Check sheet for the modelled part. Datum: model origin and axes. Units: mm. A direction names the side the tool comes from. Round coordinates to 2 decimals unless told otherwise and drop trailing zeros. Write each loop counter-clockwise with the first axis right and the second up, starting at its lowest first coordinate (ties: lowest second). Pieces come first, ordered by that corner, then holes. Notation, with made-up numbers: (4, 20.5) - (49, 20.5) arc R18 ccw to (49, 44.5) - close; hole circle Ø3 at (16.25, 84.25). An arc over 180 degrees is marked (long way). Answer as a JSON object with one key per item and string values. Group by question number.
Item 1: Release check for a two-part mould opening along X. For faces 6 (the flat face through (-25.394, 2.535, -174.72)), 7 (the flat face through (25.575, 2.636, -364.787)), 8 (the flat face through (0, -10, -289)) record: pulls with the +X half, pulls with the -X half, needs draft (parallel to the pull), parting line crosses it, or undercut.
Item 2: Set-up check for faces 1 (the flat face through (25.394, -2.535, -174.72)), 2 (the flat face through (-25.46, -2.47, -174.72)), 3 (the flat face through (25.46, 2.47, -174.72)), 4 (the flat face through (-25.575, -2.636, -364.787)), 5 (the flat face through (0, 5, -175)): record each of +Z, -Z, +X, -X, +Y, -Y from which the full face is reachable in a straight line by a thin tool's end or side.
Item 3: Gauge pin test, flat ends, axial feed: P1, Ø8, axis at y = 6.5, z = -195.5, coming from the +X side; P2, Ø4, axis at y = 0, z = -200, coming from the +X side; P3, Ø3, axis at y = 4, z = -189, coming from the +X side. Record the tip position at first contact, or that the pin passes through.
Item 4: Sectioned sample at B-B on x = -16.5. Record the boundary of the cut face in (y, z).
Item 5: Sectioned sample at D-D on y = 7.25. Record the boundary of the cut face in (x, z), plus the area to 3 significant figures.
Item 6: Sectioned sample at C-C on z = -199.5. Record the boundary of the cut face in (x, y), plus the area to 3 significant figures.
Item 7: Sectioned sample at A-A on z = -171.5. Record the boundary of the cut face in (x, y), plus the area to 3 significant figures.
Item 8: Thickness scan on line 1 (Y direction, x = 0, z = -198); line 2 (Y direction, x = 0, z = -193); line 3 (Z direction, x = 15, y = -1.75). Record the ranges inside material, lowest first.
```python
from build123d import *

# Parameters (mm, degrees)
EXTRUDE_1_DEPTH          = 18
CHAMFER_1_SIZE           = 5
CHAMFER_2_SIZE           = 5
CUT_EXTRUDE_1_DEPTH      = 8
EXTRUDE_2_REACH          = 696.741
EXTRUDE_2_END_RADIUS     = 240
EXTRUDE_3_DEPTH          = 5
EXTRUDE_4_REACH          = 929.644
EXTRUDE_4_END_RADIUS     = 232
SKETCH_10_R              = 12
CUT_EXTRUDE_7_DEPTH      = 695.872110635
CUT_EXTRUDE_7_DEPTH_BACK = 695.872110635
SKETCH_16_OUTSIDE_W      = 362.68
SKETCH_16_OUTSIDE_H      = 1204.68
SKETCH_16_OUTSIDE_W_2    = 100
SKETCH_16_OUTSIDE_H_2    = 230
SKETCH_21_R              = 1.9
CUT_EXTRUDE_17_DEPTH     = 233.862620444
SKETCH_34_OUTSIDE_W      = 120.25
SKETCH_34_OUTSIDE_H      = 70.25
CUT_EXTRUDE_18_DEPTH     = 40
CUT_EXTRUDE_19_DEPTH     = 41


with BuildPart() as part:
    # Sketch 4 → Loft 1 section 0
    with BuildSketch(Plane(origin=(0, 10, 0), x_dir=(1, 0, 0), z_dir=(0, 1, 0))):
        with BuildLine():
            Line((25, 0), (-25, 0))
            Line((-25, 0), (-25, 630))
            Line((-25, 630), (0, 672.857142857))
            Line((0, 672.857142857), (25, 630))
            Line((25, 630), (25, 0))
        make_face()
    # Sketch 1 → Loft 1 section 1
    with BuildSketch(Plane(origin=(0, 0, 0), x_dir=(1, 0, 0), z_dir=(0, 1, 0))):
        with BuildLine():
            Line((-35, 0), (35, 0))
            Line((35, 0), (35, 630))
            Line((35, 630), (0, 690))
            Line((0, 690), (-35, 630))
            Line((-35, 630), (-35, 0))
        make_face()
    loft_1 = loft()

    # Mirror 1: Loft 1 across plane
    add(loft_1.mirror(Plane.ZX))



with BuildPart() as body_2:
    # Sketch 5 → Extrude 1 (new, symmetric)
    with BuildSketch(Plane(origin=(0, 0, 0), x_dir=(1, 0, 0), z_dir=(0, 1, 0))):
        with BuildLine():
            ThreePointArc((-66.346774613, -65.189169183), (0, -55.5), (66.346774613, -65.189169183))
            ThreePointArc((66.346774613, -65.189169183), (73.061224406, -64.270510235), (76.791165228, -58.612302768))
            ThreePointArc((76.791165228, -58.612302768), (79, -30.5), (76.791165228, -2.387697232))
            ThreePointArc((76.791165228, -2.387697232), (0, -15.004503167), (-76.791165228, -2.387697232))
            ThreePointArc((-76.791165228, -2.387697232), (-79, -30.5), (-76.791165228, -58.612302768))
            ThreePointArc((-76.791165228, -58.612302768), (-73.061224406, -64.270510235), (-66.346774613, -65.189169183))
        make_face()
    extrude(amount=EXTRUDE_1_DEPTH, both=True)

    # Chamfer 1
    chamfer_1_edges = [body_2.edges().sort_by_distance(p)[0] for p in [
        (0, 18, 15.004503167),
        (-79, 18, 30.5),
        (-73.061224406, 18, 64.270510235),
        (0, 18, 55.5),
        (73.061224406, 18, 64.270510235),
        (0, -18, 55.5),
        (-73.061224406, -18, 64.270510235),
        (-79, -18, 30.5),
        (79, -18, 30.5),
        (73.061224406, -18, 64.270510235),
        (79, 18, 30.5),
    ]]
    chamfer(chamfer_1_edges, length=CHAMFER_1_SIZE)

    # Chamfer 2
    chamfer_2_edges = [body_2.edges().sort_by_distance(p)[0] for p in [
        (0, -18, 15.004503167),
    ]]
    chamfer(chamfer_2_edges, length=CHAMFER_2_SIZE)

    # Sketch 6 → Cut-Extrude 1 (cut)
    with BuildSketch(Plane(origin=(0, 18, 0), x_dir=(1, 0, 0), z_dir=(0, 1, 0))):
        with BuildLine():
            ThreePointArc((67.221840199, -55.023712607), (68.932610365, -35.286223394), (68.335500378, -15.483731767))
            ThreePointArc((68.335500378, -15.483731767), (0, -25.004503167), (-68.335500378, -15.483731767))
            ThreePointArc((-68.335500378, -15.483731767), (-68.932610365, -35.286223394), (-67.221840199, -55.023712607))
            ThreePointArc((-67.221840199, -55.023712607), (0, -45.5), (67.221840199, -55.023712607))
        make_face()
    cut_extrude_1 = extrude(amount=-CUT_EXTRUDE_1_DEPTH, mode=Mode.SUBTRACT)

    # Mirror 2: Cut-Extrude 1 across plane
    add(cut_extrude_1.mirror(Plane.ZX), mode=Mode.SUBTRACT)


with BuildPart() as part_1:
    add(part.part)

    add(body_2.part)  # Extrude 2 merges body 2
    # Extrude 2: up to this cylinder (the profile starts inside it)
    extrude_2_end = Plane(origin=(0, 0, -224.995496833), z_dir=(0, -1, 0)) * Cylinder(EXTRUDE_2_END_RADIUS, 1874.482, mode=Mode.PRIVATE)
    # Sketch 7 → Extrude 2 (add, up to the surface)
    with BuildSketch(Plane.XY, mode=Mode.PRIVATE) as extrude_2_sk1:
        Polygon((-25.828427125, 12), (-37.828427125, 0), (-25.828427125, -12), (25.828427125, -12), (37.828427125, 0), (25.828427125, 12), align=None)
    extrude_2_tool1 = extrude(extrude_2_sk1.sketch, amount=EXTRUDE_2_REACH, mode=Mode.PRIVATE) & extrude_2_end
    add(extrude_2_tool1.solids().sort_by_distance((0, 0, 0))[0])

    # Sketch 8 → Extrude 3 (add)
    with BuildSketch(Plane(origin=(0, 0, 0), x_dir=(-1, 0, 0), z_dir=(0, 0, -1))):
        Polygon((25.828427125, 12), (-25.828427125, 12), (-37.828427125, 0), (-25.828427125, -12), (25.828427125, -12), (37.828427125, 0), align=None)
    extrude(amount=EXTRUDE_3_DEPTH)



with BuildPart() as body_2_2:
    # Sketch 9 → Revolve 1 (revolve)
    with BuildSketch(Plane(origin=(0, 0, 0), x_dir=(1, 0, 0), z_dir=(0, 1, 0))):
        Polygon((0, -310), (0, -234), (-12, -234), (-22.5, -256), align=None)
    revolve(axis=Axis((0, 0, -690), (0, 0, 1)))


with BuildPart() as part_2:
    add(part_1.part)

    add(body_2_2.part)  # Extrude 4 merges body 2 2
    # Extrude 4: up to this cylinder (the profile starts inside it)
    extrude_4_end = Plane(origin=(0, 0, 287.5), z_dir=(0, -1, 0)) * Cylinder(EXTRUDE_4_END_RADIUS, 2324.288, mode=Mode.PRIVATE)
    # Sketch 10 → Extrude 4 (add, up to the surface)
    with BuildSketch(Plane(origin=(0, 0, 234), x_dir=(-1, 0, 0), z_dir=(0, 0, -1)), mode=Mode.PRIVATE) as extrude_4_sk1:
        with Locations(Location((0, 0, 0), (0, 0, 90))):
            Circle(SKETCH_10_R)
    extrude_4_tool1 = extrude(extrude_4_sk1.sketch, amount=EXTRUDE_4_REACH, mode=Mode.PRIVATE) & extrude_4_end
    add(extrude_4_tool1.solids().sort_by_distance((0, 0, 234))[0])

    # Sketch 16 outside → Cut-Extrude 7 (cut, two sides: drawn at the far end of the back side and taken through both)
    with BuildSketch(Plane(origin=(0, 0, 0), x_dir=(1, 0, 0), z_dir=(0, 1, 0)).offset(-CUT_EXTRUDE_7_DEPTH_BACK)):
        with Locations((0, 190)):
            Rectangle(SKETCH_16_OUTSIDE_W, SKETCH_16_OUTSIDE_H)
        with Locations((0, 270)):
            Rectangle(SKETCH_16_OUTSIDE_W_2, SKETCH_16_OUTSIDE_H_2, mode=Mode.SUBTRACT)
    extrude(amount=CUT_EXTRUDE_7_DEPTH + CUT_EXTRUDE_7_DEPTH_BACK, mode=Mode.SUBTRACT)

    # Sketch 21 → Cut-Extrude 17 (cut, through all)
    with BuildSketch(Plane.XY.offset(-155)):
        Circle(SKETCH_21_R)
    extrude(amount=-CUT_EXTRUDE_17_DEPTH, mode=Mode.SUBTRACT)

    # Sketch 34 outside → Cut-Extrude 18 (cut)
    with BuildSketch(Plane.XY.offset(-155)):
        Rectangle(SKETCH_34_OUTSIDE_W, SKETCH_34_OUTSIDE_H)
        Polygon((-22.928932188, -5), (22.928932188, -5), (27.928932188, 0), (22.928932188, 5), (-22.928932188, 5), (-27.928932188, 0), align=None, mode=Mode.SUBTRACT)
    extrude(amount=-CUT_EXTRUDE_18_DEPTH, mode=Mode.SUBTRACT)

    # Sketch 35 → Cut-Extrude 19 (cut)
    with BuildSketch(Plane(origin=(0, 0, -385), x_dir=(-1, 0, 0), z_dir=(0, 0, -1))):
        Polygon((-28.211774901, 0), (-23.011774901, -5.2), (23.011774901, -5.2), (28.211774901, 0), (23.011774901, 5.2), (-23.011774901, 5.2), align=None)
    extrude(amount=-CUT_EXTRUDE_19_DEPTH, mode=Mode.SUBTRACT)


solid = part_2.part
```
Completed:
{
 "1": {"face 6": "pulls with the -X half", "face 7": "undercut", "face 8": "needs draft"},
 "2": {"face 1": "+Z, +X, -Y", "face 2": "+Z, -X, -Y", "face 3": "+Z, +X, +Y", "face 4": "-Z", "face 5": "+Z, +X, -X, +Y"},
 "3": {"P1": "x = 32.5", "P2": "x = 35", "P3": "x = 25.43"},
 "4": {"outline": "(-10, -385) - (-5.2, -385) - (-5.2, -344) - (5.2, -344) - (5.2, -385) - (10, -385) - (10, -195) - (5, -195) - (5, -155) - (-5, -155) - (-5, -195) - (-10, -195) - close"},
 "5": {"outline": "(-27.75, -385) - (27.75, -385) - (27.75, -195) - (-27.75, -195) - close", "area": "10,500 mm²"},
 "6": {"outline": "(-35, 0) - (-25, -10) - (25, -10) - (35, 0) - (25, 10) - (-25, 10) - close; hole circle Ø3.8 at (0, 0)", "area": "1,190 mm²"},
 "7": {"outline": "(-27.93, 0) - (-22.93, -5) - (22.93, -5) - (27.93, 0) - (22.93, 5) - (-22.93, 5) - close; hole circle Ø3.8 at (0, 0)", "area": "497 mm²"},
 "8": {"line 1": "-10 to -1.9, 1.9 to 10", "line 2": "-5 to -1.9, 1.9 to 5", "line 3": "-344 to -155"}
}
